from build123d import *

# Parameters (mm, degrees)
CUT_EXTRUDE1_DEPTH = 30.593736097


with BuildPart() as part:
    # Sketch1 → Revolve1 (revolve)
    with BuildSketch(Plane(origin=(0, 0, 0), x_dir=(0, 0, -1), z_dir=(1, 0, 0)), mode=Mode.PRIVATE) as revolve1_sk:
        Polygon((0, 0), (23.5204, 0), (23.5204, 8.286019513), (23.5204, 12.7), (0, 12.7), (0, 8.286019513), align=None)
    revolve(revolve1_sk.sketch.rotate(Axis((0, 0, 0), (0, 0, -1)), 180), axis=Axis((0, 0, 0), (0, 0, -1)))

    # Sketch2 → Cut-Extrude1 (cut, through all)
    with BuildSketch(Plane.XY):
        Polygon((3.666174209, 6.35), (-3.666174209, 6.35), (-7.332348419, 0), (-3.666174209, -6.35), (3.666174209, -6.35), (7.332348419, 0), align=None)
    extrude(amount=-CUT_EXTRUDE1_DEPTH, mode=Mode.SUBTRACT)


solid = part.part
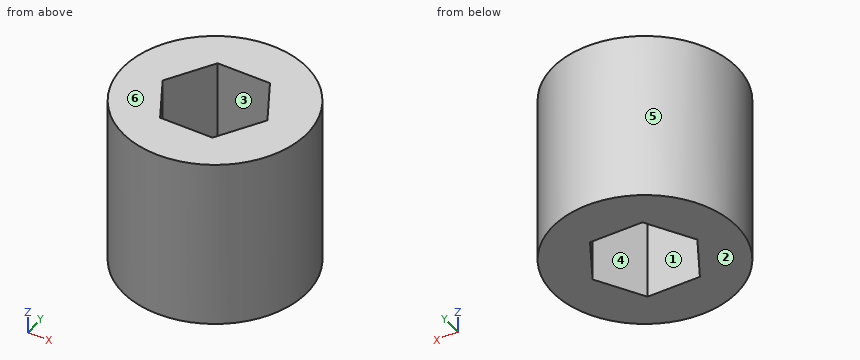
Verification items for the finished model (mm, model axes). Face numbers are marked on the shaded views. A direction names the side the tool comes from. Give positions to 0.01 mm unless a question says otherwise; leave off trailing zeros. Write each loop counter-clockwise with the first axis right and the second up, starting at its lowest first coordinate (ties: lowest second). Pieces come first, ordered by that corner, then holes. Notation, with made-up numbers: M 73.5,89 L 83.5,89 A23 cw 83.5,120 Z; hole C 21.25,89.25 d1. An arc over 180 degrees is marked long. Use CSV: the item, a comma, the result in double quotes.
1) Cross-section at A-A (x = 0). Enter the section's corners in (y, z).
Final values:
outline,"M -12.7,-23.52 L -6.35,-23.52 L -6.35,0 L -12.7,0 Z; M 6.35,-23.52 L 12.7,-23.52 L 12.7,0 L 6.35,0 Z"
2) Release check for a two-part mould opening along X. For the marked faces 3, 4, 5 and 6 record: released by +X, released by -X, zero draft, split by the parting line, or undercut.
Final values:
face 3,"undercut"
face 4,"undercut"
face 5,"split by the parting line"
face 6,"zero draft"
3) Cross-section at D-D (y = 8.75). Enter the section's corners in (x, z), plus the area to 3 significant figures.
Final values:
outline,"M -9.2,-23.52 L 9.2,-23.52 L 9.2,0 L -9.2,0 Z"
area,"433 mm²"
4) Material ranges on line 1 along Y through (x, z) = (-2.5, -22.5); line 2 along Y through (x, z) = (6.5, -12.5); line 3 along X through (y, z) = (-3.5, -19.5), recorded low to high.
Final values:
line 1,"-12.45 to -6.35, 6.35 to 12.45"
line 2,"-10.91 to -1.44, 1.44 to 10.91"
line 3,"-12.21 to -5.31, 5.31 to 12.21"
5) Cross-section at C-C (z = -9). Enter the section's corners in (x, y), plus the area to 3 significant figures.
Final values:
outline,"C 0,0 d25.4; hole M -7.33,0 L -3.67,-6.35 L 3.67,-6.35 L 7.33,0 L 3.67,6.35 L -3.67,6.35 Z"
area,"367 mm²"
6) Access from +Z, -Z, +X, -X, +Y, -Y to the whole of each face (thin tool, end or side, straight path). Record for the marked faces 1 and 2.
Final values:
face 1,"+Z, -Z"
face 2,"-Z, +X, -X, +Y, -Y"
7) Cross-section at B-B (y = 5.75). Enter the section's corners in (x, z), plus the area to 3 significant figures.
Final values:
outline,"M -11.32,-23.52 L -4.01,-23.52 L -4.01,0 L -11.32,0 Z; M 4.01,-23.52 L 11.32,-23.52 L 11.32,0 L 4.01,0 Z"
area,"344 mm²"
8) Go/stop test with flat-tipped pins: pin 1 Ø4 at (x, z) = (5.5, -12) entering from +Y; pin 2 Ø1.5 at (x, z) = (8, -12) entering from +Y; pin 3 Ø5 at (x, z) = (-10, -7.5) entering from +Y; pin 4 Ø3.5 at (x, z) = (-1, -9) entering from +Y. Record where each tip stops, or that it passes through.
Final values:
pin 1,"y = 12.21"
pin 2,"y = 10.43"
pin 3,"y = 10.25"
pin 4,"y = 12.7"
